Read the model definition and answer for the solid it produces. Units are mm, in the model's axes. Face numbers are marked on the shaded views. Give positions to 0.01 mm unless a question says otherwise; leave off trailing zeros. Order: outer loops, then holes, each group sorted by start corner. A loop starts at its lowest first (then second) coordinate and runs counter-clockwise, first axis right, second up.
```python
from build123d import *

# Parameters (mm, degrees)
ESQUISSE1_W             = 50
ESQUISSE1_H             = 10
BOSS_EXTRU_1_DEPTH      = 10
ENL_V_MAT_EXTRU_1_REACH = 53.962
ESQUISSE2_R             = 2.5


with BuildPart() as part:
    # Esquisse1 → Boss.-Extru.1 (new body)
    with BuildSketch(Plane.XY):
        with Locations((25, 5)):
            Rectangle(ESQUISSE1_W, ESQUISSE1_H)
    extrude(amount=BOSS_EXTRU_1_DEPTH)

    # Esquisse2 → Enlèv. mat.-Extru.1 (cut, up to next)
    with BuildSketch(Plane.XY.offset(10), mode=Mode.PRIVATE) as enl_v_mat_extru_1_sk1:
        with Locations((5, 5)):
            Circle(ESQUISSE2_R)
    enl_v_mat_extru_1_tool1 = extrude(enl_v_mat_extru_1_sk1.sketch, amount=-ENL_V_MAT_EXTRU_1_REACH, mode=Mode.PRIVATE) & part.part
    # Esquisse2 → Enlèv. mat.-Extru.1 (cut, up to next)
    with BuildSketch(Plane.XY.offset(10), mode=Mode.PRIVATE) as enl_v_mat_extru_1_sk2:
        with Locations((15, 5)):
            Circle(ESQUISSE2_R)
    enl_v_mat_extru_1_tool2 = extrude(enl_v_mat_extru_1_sk2.sketch, amount=-ENL_V_MAT_EXTRU_1_REACH, mode=Mode.PRIVATE) & part.part
    # Esquisse2 → Enlèv. mat.-Extru.1 (cut, up to next)
    with BuildSketch(Plane.XY.offset(10), mode=Mode.PRIVATE) as enl_v_mat_extru_1_sk3:
        with Locations((25, 5)):
            Circle(ESQUISSE2_R)
    enl_v_mat_extru_1_tool3 = extrude(enl_v_mat_extru_1_sk3.sketch, amount=-ENL_V_MAT_EXTRU_1_REACH, mode=Mode.PRIVATE) & part.part
    # Esquisse2 → Enlèv. mat.-Extru.1 (cut, up to next)
    with BuildSketch(Plane.XY.offset(10), mode=Mode.PRIVATE) as enl_v_mat_extru_1_sk4:
        with Locations((35, 5)):
            Circle(ESQUISSE2_R)
    enl_v_mat_extru_1_tool4 = extrude(enl_v_mat_extru_1_sk4.sketch, amount=-ENL_V_MAT_EXTRU_1_REACH, mode=Mode.PRIVATE) & part.part
    # Esquisse2 → Enlèv. mat.-Extru.1 (cut, up to next)
    with BuildSketch(Plane.XY.offset(10), mode=Mode.PRIVATE) as enl_v_mat_extru_1_sk5:
        with Locations((45, 5)):
            Circle(ESQUISSE2_R)
    enl_v_mat_extru_1_tool5 = extrude(enl_v_mat_extru_1_sk5.sketch, amount=-ENL_V_MAT_EXTRU_1_REACH, mode=Mode.PRIVATE) & part.part
    add(enl_v_mat_extru_1_tool1.solids().sort_by_distance((5, 5, 10))[0], mode=Mode.SUBTRACT)
    add(enl_v_mat_extru_1_tool2.solids().sort_by_distance((15, 5, 10))[0], mode=Mode.SUBTRACT)
    add(enl_v_mat_extru_1_tool3.solids().sort_by_distance((25, 5, 10))[0], mode=Mode.SUBTRACT)
    add(enl_v_mat_extru_1_tool4.solids().sort_by_distance((35, 5, 10))[0], mode=Mode.SUBTRACT)
    add(enl_v_mat_extru_1_tool5.solids().sort_by_distance((45, 5, 10))[0], mode=Mode.SUBTRACT)


solid = part.part
```
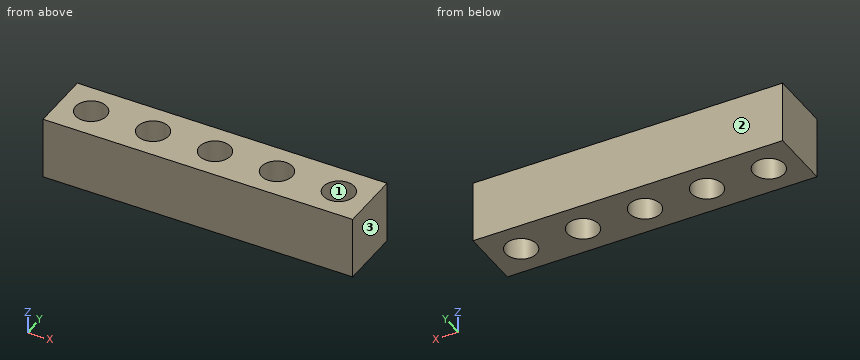
1) The part is cut by section B-B on y = 5. Determine the outline of the cut face in (x, z), and give its area (3 significant figures).
Final values:
outline: (0, 0) - (2.5, 0) - (2.5, 10) - (0, 10) - close; (7.5, 0) - (12.5, 0) - (12.5, 10) - (7.5, 10) - close; (17.5, 0) - (22.5, 0) - (22.5, 10) - (17.5, 10) - close; (27.5, 0) - (32.5, 0) - (32.5, 10) - (27.5, 10) - close; (37.5, 0) - (42.5, 0) - (42.5, 10) - (37.5, 10) - close; (47.5, 0) - (50, 0) - (50, 10) - (47.5, 10) - close
area: 250 mm2
2) For a pull along Y with two mould halves and no side action, classify the marked faces 1, 2 and 3 as released by +Y, released by -Y, zero draft, split by the parting line, or undercut.
Final values:
face 1: undercut
face 2: released by +Y
face 3: zero draft
3) The part is cut by section C-C on z = 6.25. Determine the outline of the cut face in (x, y), and give its area (3 significant figures).
Final values:
outline: (0, 0) - (50, 0) - (50, 10) - (0, 10) - close; hole circle Ø5 at (5, 5); hole circle Ø5 at (15, 5); hole circle Ø5 at (25, 5); hole circle Ø5 at (35, 5); hole circle Ø5 at (45, 5)
area: 402 mm2
4) Given pin 1 (4.5 mm diameter, centred on x = 25, y = 5, fed in from -Z); pin 2 (1 mm diameter, centred on x = 41.5, z = 3, fed in from -Y), each flat-ended and moving along its own axis, determine where each tip first touches the part or whether it passes through.
Final values:
pin 1: passes through
pin 2: stops at y = 0
5) The part is cut by section A-A on x = 5. Determine the outline of the cut face in (y, z), and give its area (3 significant figures).
Final values:
outline: (0, 0) - (2.5, 0) - (2.5, 10) - (0, 10) - close; (7.5, 0) - (10, 0) - (10, 10) - (7.5, 10) - close
area: 50.0 mm2
6) Consider L1, parallel to X at y = 4.5, z = 4.25; L2, parallel to Y at x = 5, z = 2.75; L3, parallel to X at y = 4.75, z = 6.5. Determine where each line is inside the solid, lowest interval first.
Final values:
L1: x = 0 to 2.55, 7.45 to 12.55, 17.45 to 22.55, 27.45 to 32.55, 37.45 to 42.55, 47.45 to 50
L2: y = 0 to 2.5, 7.5 to 10
L3: x = 0 to 2.51, 7.49 to 12.51, 17.49 to 22.51, 27.49 to 32.51, 37.49 to 42.51, 47.49 to 50
